The listing builds one solid part. Answer for the finished solid, in the listing's coordinates (mm). Face numbers are marked on the shaded views. A direction names the side the tool comes from. Round coordinates to 2 decimals unless told otherwise and drop trailing zeros. Write each loop counter-clockwise with the first axis right and the second up, starting at its lowest first coordinate (ties: lowest second). Pieces come first, ordered by that corner, then holes.
Item 1: A tool of negligible diameter and unlimited length cuts with its end or side. For the marked faces 4, 5, 6 and 7, from which of +Z, -Z, +X, -X, +Y, -Y can it reach the whole face along a straight path? Write none if from no direction.
Item 2: Each of these flat-tipped pins is pushed along its axis until it touches: pin 1 (4 mm diameter, centred on x = 13, z = 11.5, fed in from -Y); pin 2 (3 mm diameter, centred on y = 67, z = 13.5, fed in from -X); pin 3 (1 mm diameter, centred on y = 60.5, z = 13.5, fed in from -X); pin 4 (8 mm diameter, centred on y = 62, z = 6.5, fed in from +X). Where does it stop, or does it pass through?
Item 3: For a pull along Z with two mould halves and no side action, classify the marked faces 1, 2 and 3 as +Z half, -Z half, draft (parallel to the pull), parting line (faces both ways), or undercut.
Item 4: Find section D-D on y = 56. Give the vertices of the cut face in (x, z).
Item 5: Find section B-B on x = -1.65. Give the vertices of the cut face in (y, z), then the cut area to 3 significant figures.
Item 6: Find section C-C on z = 3. Give the vertices of the cut face in (x, y).
Item 7: Find section A-A on z = 7.75. Give the vertices of the cut face in (x, y), then the cut area to 3 significant figures.
Item 8: Find the intervals of material crossed by probe 1 along Y at (x, z) = (4.5, 10); probe 2 along X at (y, z) = (14.25, 7.75); probe 3 along Y at (x, z) = (-23, 8.25), in increasing order.
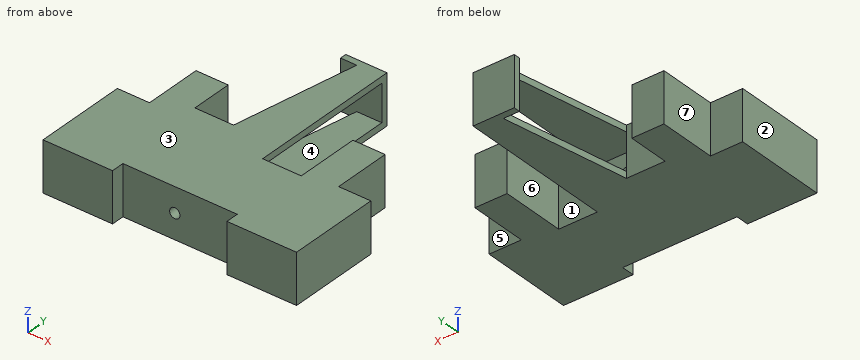
```python
from build123d import *

# Parameters (mm, degrees)
BOSS_EXTRU_1_DEPTH      = 15.5
ENL_V_START             = -2
ESQUISSE2_W             = 17.606783298
ESQUISSE2_H             = 46.2
ENL_V_MAT_EXTRU_1_DEPTH = 11.5
ENL_V_MAT_EXTRU_2_REACH = 88.103
ESQUISSE3_R             = 1.6


with BuildPart() as part:
    # Esquisse1 → Boss.-Extru.1 (new body)
    with BuildSketch(Plane.XY):
        Polygon((-39.35, 0), (-39.35, 28.8), (-29.35, 28.8), (-29.35, 46.8), (-19.35, 46.8), (-19.35, 33.9), (-7.35, 33.9), (-0.455615054, 73), (-5.455615054, 73), (-5.455615054, 75), (7.35, 75), (7.35, 26.8), (19.35, 26.8), (19.35, 46.8), (29.35, 46.8), (29.35, 28.8), (39.35, 28.8), (39.35, 0), (17.75, 0), (17.75, 4), (-17.75, 4), (-17.75, 0), align=None)
    extrude(amount=BOSS_EXTRU_1_DEPTH)

    # Esquisse2 → Enlèv. mat.-Extru.1 (cut)
    with BuildSketch(Plane.XY.offset(15.5).offset(ENL_V_START)):
        with Locations((1.453391649, 49.9)):
            Rectangle(ESQUISSE2_W, ESQUISSE2_H)
    extrude(amount=-ENL_V_MAT_EXTRU_1_DEPTH, mode=Mode.SUBTRACT)

    # Esquisse3 → Enlèv. mat.-Extru.2 (cut, up to next)
    with BuildSketch(Plane.XZ, mode=Mode.PRIVATE) as enl_v_mat_extru_2_sk1:
        with Locations(Location((-1.65, 7.75, 0), (0, 0, 270))):
            Circle(ESQUISSE3_R)
    enl_v_mat_extru_2_tool1 = extrude(enl_v_mat_extru_2_sk1.sketch, amount=-ENL_V_MAT_EXTRU_2_REACH, mode=Mode.PRIVATE) & part.part
    add(enl_v_mat_extru_2_tool1.solids().sort_by_distance((-1.65, 0, 7.75))[0], mode=Mode.SUBTRACT)


solid = part.part
```
Check values:
1. face 4: none
1. face 5: +Z, -Z, +X, +Y
1. face 6: +Z, -Z, +Y
1. face 7: +Z, -Z, -X, +Y
2. pin 1: stops at y = 4
2. pin 2: stops at x = -1.78
2. pin 3: stops at x = -2.75
2. pin 4: passes through
3. face 1: undercut
3. face 2: draft
3. face 3: +Z half
4. outline: (-3.45, 0) - (7.35, 0) - (7.35, 2) - (-3.45, 2) - close; (-3.45, 13.5) - (7.35, 13.5) - (7.35, 15.5) - (-3.45, 15.5) - close
5. outline: (4, 0) - (66.23, 0) - (66.23, 2) - (26.8, 2) - (26.8, 6.15) - (4, 6.15) - close; (4, 9.35) - (26.8, 9.35) - (26.8, 13.5) - (66.23, 13.5) - (66.23, 15.5) - (4, 15.5) - close; (73, 0) - (75, 0) - (75, 15.5) - (73, 15.5) - close
5. area: 469 mm2
6. outline: (-39.35, 0) - (-17.75, 0) - (-17.75, 4) - (17.75, 4) - (17.75, 0) - (39.35, 0) - (39.35, 28.8) - (29.35, 28.8) - (29.35, 46.8) - (19.35, 46.8) - (19.35, 26.8) - (-7.35, 26.8) - (-7.35, 33.9) - (-19.35, 33.9) - (-19.35, 46.8) - (-29.35, 46.8) - (-29.35, 28.8) - (-39.35, 28.8) - close; (-5.46, 73) - (7.35, 73) - (7.35, 75) - (-5.46, 75) - close
7. outline: (-39.35, 0) - (-17.75, 0) - (-17.75, 4) - (-3.25, 4) - (-3.25, 26.8) - (-7.35, 26.8) - (-7.35, 33.9) - (-19.35, 33.9) - (-19.35, 46.8) - (-29.35, 46.8) - (-29.35, 28.8) - (-39.35, 28.8) - close; (-5.46, 73) - (7.35, 73) - (7.35, 75) - (-5.46, 75) - close; (-0.05, 4) - (17.75, 4) - (17.75, 0) - (39.35, 0) - (39.35, 28.8) - (29.35, 28.8) - (29.35, 46.8) - (19.35, 46.8) - (19.35, 26.8) - (-0.05, 26.8) - close
7. area: 2,450 mm2
8. probe 1: y = 4 to 26.8, 73 to 75
8. probe 2: x = -39.35 to -3.25, -0.05 to 39.35
8. probe 3: y = 0 to 46.8
